from build123d import *

# Parameters (mm, degrees)
SKETCH1_R           = 1.6
BOSS_EXTRUDE1_DEPTH = 10


with BuildPart() as part:
    # Sketch1 → Boss-Extrude1 (new body)
    with BuildSketch(Plane.XY):
        with BuildLine():
            Line((0, -1), (40, -1))
            ThreePointArc((40, -1), (40.707106781, -0.707106781), (41, 0))
            Line((41, 0), (41, 40))
            ThreePointArc((41, 40), (40.707106781, 40.707106781), (40, 41))
            Line((40, 41), (0, 41))
            ThreePointArc((0, 41), (-0.707106781, 40.707106781), (-1, 40))
            Line((-1, 40), (-1, 0))
            ThreePointArc((-1, 0), (-0.707106781, -0.707106781), (0, -1))
        make_face()
        with Locations((4, 36)):
            Circle(SKETCH1_R, mode=Mode.SUBTRACT)
        with Locations((36, 36)):
            Circle(SKETCH1_R, mode=Mode.SUBTRACT)
        with Locations((36, 4)):
            Circle(SKETCH1_R, mode=Mode.SUBTRACT)
        with Locations((4, 4)):
            Circle(SKETCH1_R, mode=Mode.SUBTRACT)
        with BuildLine():
            Line((36, 8), (37.5, 8))
            ThreePointArc((37.5, 8), (38.207106781, 8.292893219), (38.5, 9))
            Line((38.5, 9), (38.5, 31))
            ThreePointArc((38.5, 31), (38.207106781, 31.707106781), (37.5, 32))
            Line((37.5, 32), (36, 32))
            ThreePointArc((36, 32), (33.171572875, 33.171572875), (32, 36))
            Line((32, 36), (32, 37.5))
            ThreePointArc((32, 37.5), (31.707106781, 38.207106781), (31, 38.5))
            Line((31, 38.5), (9, 38.5))
            ThreePointArc((9, 38.5), (8.292893219, 38.207106781), (8, 37.5))
            Line((8, 37.5), (8, 36))
            ThreePointArc((8, 36), (6.828427125, 33.171572875), (4, 32))
            Line((4, 32), (2.5, 32))
            ThreePointArc((2.5, 32), (1.792893219, 31.707106781), (1.5, 31))
            Line((1.5, 31), (1.5, 9))
            ThreePointArc((1.5, 9), (1.792893219, 8.292893219), (2.5, 8))
            Line((2.5, 8), (4, 8))
            ThreePointArc((4, 8), (6.828427125, 6.828427125), (8, 4))
            Line((8, 4), (8, 2.5))
            ThreePointArc((8, 2.5), (8.292893219, 1.792893219), (9, 1.5))
            Line((9, 1.5), (31, 1.5))
            ThreePointArc((31, 1.5), (31.707106781, 1.792893219), (32, 2.5))
            Line((32, 2.5), (32, 4))
            ThreePointArc((32, 4), (33.171572875, 6.828427125), (36, 8))
        make_face(mode=Mode.SUBTRACT)
    extrude(amount=BOSS_EXTRUDE1_DEPTH)


solid = part.part
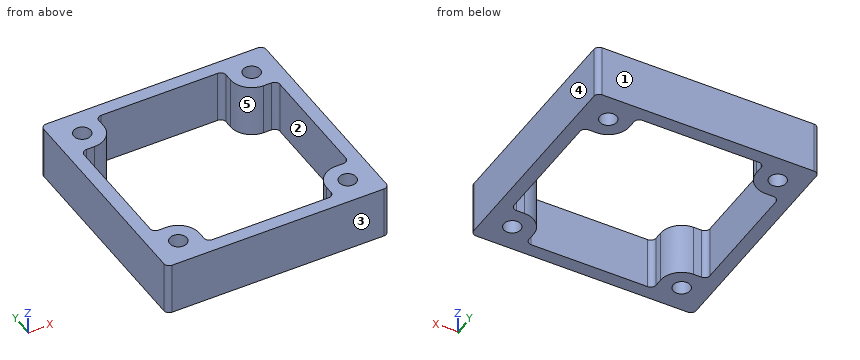
Part model, mm, in its own coordinate system. Face numbers are marked on the shaded views. A direction names the side the tool comes from. Give positions to 0.01 mm unless a question says otherwise; leave off trailing zeros. Loops run counter-clockwise (first coordinate to the right, second up) from the corner with the lowest first, then second, coordinate; pieces in that order, holes last. Notation, with made-up numbers: (-13.5, 51) -> (-5.5, 51) arc R31 cw to (-5.5, 88) -> close; hole circle Ø11 at (80, 23.5). An arc over 180 degrees is marked (long way). Write each question's results on one line, items separated by ' | '. Start each with the question number.
Q1. Band-saw the part on C-C on z = 7.25. Count the separate pieces of the cut face and the enclosed holes in it, plus the area to 3 significant figures.
Q2. Band-saw the part on A-A on x = 27. List the corners of the cut face in (y, z).
Q3. Band-saw the part on D-D on y = 3.5. List the corners of the cut face in (x, z), plus the area to 3 significant figures.
Q4. Wall check: L1, parallel to Y at x = 4, z = 4.75; L2, parallel to Y at x = 27, z = 5.75. Give the ranges that are in metal, low to high.
Q5. Which spindle directions (+Z, -Z, +X, -X, +Y, -Y) get a long thin tool onto all of the face, cutting with end or side? Do the marked faces 1 and 2. Say none if no direction does.
Q6. Pull direction Y, two halves, no side cores. Call the marked faces 3, 4 and 5: +Y half, -Y half, draft (parallel to the pull), parting line (faces both ways), or undercut.
Q7. Pin check, flat tips, straight feed: P1, Ø3, axis at x = 4, y = 4, coming from the +Z side; P2, Ø4, axis at x = 4, y = 36, coming from the +Z side. Stop position of each tip, or through.
Results are:
1) separate pieces: 1 | enclosed holes: 5 | area: 519 mm²
2) outline: (-1, 0) -> (1.5, 0) -> (1.5, 10) -> (-1, 10) -> close; (38.5, 0) -> (41, 0) -> (41, 10) -> (38.5, 10) -> close
3) outline: (-1, 0) -> (2.48, 0) -> (2.48, 10) -> (-1, 10) -> close; (5.52, 0) -> (8, 0) -> (8, 10) -> (5.52, 10) -> close; (32, 0) -> (34.48, 0) -> (34.48, 10) -> (32, 10) -> close; (37.52, 0) -> (41, 0) -> (41, 10) -> (37.52, 10) -> close | area: 119 mm²
4) L1: y = -1 to 2.4, 5.6 to 8, 32 to 34.4, 37.6 to 41 | L2: y = -1 to 1.5, 38.5 to 41
5) face 1: +Z, -Z, +X, -X, +Y | face 2: +Z, -Z
6) face 3: -Y half | face 4: draft | face 5: undercut
7) P1: passes through | P2: stops at z = 10
